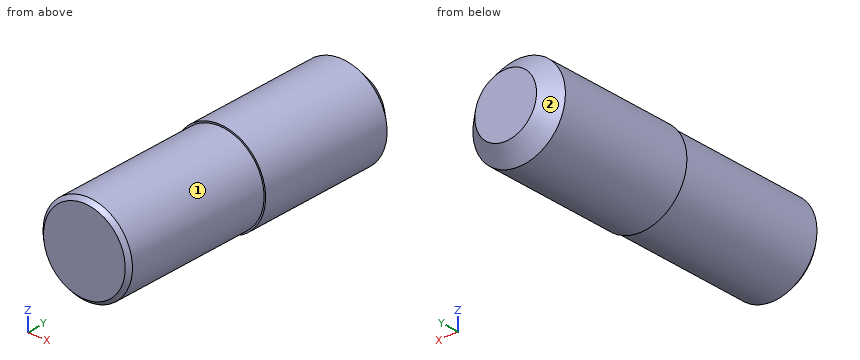
Autodesk Inventor part; units mm, degrees
ref_plane "YZ Plane" through (0, 0, 0) normal (1, 0, 0) x (0, 1, 0)
ref_plane "XZ Plane" through (0, 0, 0) normal (0, 1, 0) x (-1, 0, 0)
ref_plane "XY Plane" through (0, 0, 0) normal (0, 0, 1) x (1, 0, 0)
sketch "Esboço1" plane through (0, 0, 0) normal (0, 0, 1) x (1, 0, 0)
  line L0 (-3.6, 0) -> (0.6, 0) construction
  line L1 (0, -14) -> (0, 14) construction
  line L2 (-3, 10) -> (0, 10)
  line L3 (0, 10) -> (0, -10)
  line L4 (0, -10) -> (-3, -10)
  line L5 (-3, -10) -> (-3, 10)
  line L6 (-3, 0) -> (-2.9, 0)
  line L7 (-2.9, 0) -> (-2.9, -10)
  line L8 (-2, 10) -> (-3, 9)
  line L9 (-2.9, -9.75) -> (-2.65, -10)
  line L10 (-3, 0.25) -> (-2.9, 0.15)
  point P0 (0, 0)
  point P1 (-2.75, 0)
  dimension "d0" = 6
  dimension "d1" = 5.8
  dimension "d2" = 10
  dimension "d3" = 20
  dimension "d4" = 1
  dimension "d5" = 1
  dimension "d6" = 0.25
  dimension "d7" = 0.25
  dimension "d8" = 45
  dimension "d12" = 0.25
revolve "Revolução1" add sketch "Esboço1" angle 360 about axis through (0, 10, 0) along (0, -1, 0) contours L2 L3 L4 L9 L7 L6 L5 L8
thread "Rosca1"
equation "\"d6\" = d7"
properties part number "GRJ-03-118" material "Aço SAE 1045"
Input: part model. Units: mm. Frame: model coordinates. Face numbers are marked on the shaded views. A direction names the side the tool comes from. Round coordinates to 2 decimals unless told otherwise and drop trailing zeros. Loops run counter-clockwise (first coordinate to the right, second up) from the corner with the lowest first, then second, coordinate; pieces in that order, holes last. Notation, with made-up numbers: (78, -37.75) -> (136, -37.75) arc R30 cw to (136, -10.75) -> close; hole circle Ø11 at (31.5, -30). An arc over 180 degrees is marked (long way). Write each question's results on one line, items separated by ' | '.
1. Section C-C (y = -4.75). Return loops of the section in (x, z), and give its area (3 significant figures).
Geometry results:
outline: circle Ø5.8 at (0, 0) | area: 26.4 mm2
2. Set-up query: the marked faces 1 and 2. Return all of +Z, -Z, +X, -X, +Y, -Y with unobstructed straight access to the full face (end or side cutting, diameter ignored); none if empty.
Geometry results:
face 1: -Y | face 2: +Y
3. Section B-B (x = 0). Return loops of the section in (y, z), and give its area (3 significant figures).
Geometry results:
outline: (-10, -2.65) -> (-9.75, -2.9) -> (0, -2.9) -> (0, -3) -> (9, -3) -> (10, -2) -> (10, 2) -> (9, 3) -> (0, 3) -> (0, 2.9) -> (-9.75, 2.9) -> (-10, 2.65) -> close | area: 117 mm2
4. Section D-D (y = 7). Return loops of the section in (x, z).
Geometry results:
outline: circle Ø6 at (0, 0)
5. First-contact query: P1, Ø2, axis at y = -4, z = 2, coming from the -X side; P2, Ø3, axis at y = -3, z = 0, coming from the -X side. Flat tips, straight axial feed; report the tip coordinate or a pass-through.
Geometry results:
P1: x = -2.72 | P2: x = -2.9
6. Ray query, line 1 (Z direction, x = 0.05, y = -3); line 2 (X direction, y = 8, z = 2.35); line 3 (Y direction, x = -0.55, z = -2). Return the intervals inside material, ascending. Write a range as from..to.
Geometry results:
line 1: -2.9..2.9 | line 2: -1.86..1.86 | line 3: -10..9.93
7. Section A-A (z = 0). Return loops of the section in (x, y).
Geometry results:
outline: (-3, 0) -> (-2.9, 0) -> (-2.9, -9.75) -> (-2.65, -10) -> (2.65, -10) -> (2.9, -9.75) -> (2.9, 0) -> (3, 0) -> (3, 9) -> (2, 10) -> (-2, 10) -> (-3, 9) -> close
